CAD build for the part. Positions are in the model's coordinates, mm. A direction names the side the tool comes from. Coordinates: 2 decimals unless noted, no trailing zeros. Loops run counter-clockwise (first coordinate to the right, second up) from the corner with the lowest first, then second, coordinate; pieces in that order, holes last. Notation, with made-up numbers: (-13, 41) -> (6, 41) arc R13 cw to (6, 56) -> close; hole circle Ø8 at (9.5, 40.25). An arc over 180 degrees is marked (long way). Answer as CSV lines item,"result". Start each with the question number.
from build123d import *

# Parameters (mm, degrees)
SKETCH1_R             = 1
BOSS_EXTRUDE1_DEPTH   = 8
BOSS_EXTRUDE1_2_DEPTH = 8
BOSS_EXTRUDE1_3_DEPTH = 8
BOSS_EXTRUDE1_4_DEPTH = 8
SKETCH2_R             = 1.75
BOSS_EXTRUDE2_DEPTH   = 6
SKETCH3_W             = 99
SKETCH3_H             = 63
BOSS_EXTRUDE3_DEPTH   = 2
FILLET1_R             = 2
BOSS_EXTRUDE4_START   = 8
BOSS_EXTRUDE4_DEPTH   = 8
CUT_EXTRUDE1_REACH    = 106.833
SKETCH6_W             = 18
SKETCH6_H             = 7
CUT_EXTRUDE2_REACH    = 83.514
SKETCH8_W             = 18
SKETCH8_H             = 7


with BuildPart() as part:
    # Sketch1 → Boss-Extrude1 (new body)
    with BuildSketch(Plane(origin=(0, 0, 0), x_dir=(1, 0, 0), z_dir=(0, 1, 0))):
        with Locations(Location((-33.5, 25, 0), (0, 0, 270))):
            Circle(SKETCH1_R)
    extrude(amount=BOSS_EXTRUDE1_DEPTH)



with BuildPart() as body_2:
    # Sketch1 → Boss-Extrude1 2 (new body)
    with BuildSketch(Plane(origin=(0, 0, 0), x_dir=(1, 0, 0), z_dir=(0, 1, 0))):
        with Locations(Location((33.5, 25, 0), (0, 0, 270))):
            Circle(SKETCH1_R)
    extrude(amount=BOSS_EXTRUDE1_2_DEPTH)


with BuildPart() as body_3:
    # Sketch1 → Boss-Extrude1 3 (new body)
    with BuildSketch(Plane(origin=(0, 0, 0), x_dir=(1, 0, 0), z_dir=(0, 1, 0))):
        with Locations(Location((-45.75, -25, 0), (0, 0, 270))):
            Circle(SKETCH1_R)
    extrude(amount=BOSS_EXTRUDE1_3_DEPTH)


with BuildPart() as body_4:
    # Sketch1 → Boss-Extrude1 4 (new body)
    with BuildSketch(Plane(origin=(0, 0, 0), x_dir=(1, 0, 0), z_dir=(0, 1, 0))):
        with Locations(Location((43.25, -25, 0), (0, 0, 270))):
            Circle(SKETCH1_R)
    extrude(amount=BOSS_EXTRUDE1_4_DEPTH)


with BuildPart() as part_1:
    add(part.part)

    add(body_2.part)  # Boss-Extrude2 merges body 2

    add(body_3.part)  # Boss-Extrude2 merges body 3

    add(body_4.part)  # Boss-Extrude2 merges body 4
    # Sketch2 → Boss-Extrude2 (add)
    with BuildSketch(Plane(origin=(0, 0, 0), x_dir=(1, 0, 0), z_dir=(0, 1, 0))):
        with Locations(Location((-33.5, 25, 0), (0, 0, 270))):
            Circle(SKETCH2_R)
        with Locations(Location((33.5, 25, 0), (0, 0, 270))):
            Circle(SKETCH2_R)
        with Locations(Location((43.25, -25, 0), (0, 0, 270))):
            Circle(SKETCH2_R)
        with Locations(Location((-45.75, -25, 0), (0, 0, 270))):
            Circle(SKETCH2_R)
    extrude(amount=BOSS_EXTRUDE2_DEPTH)

    # Sketch3 → Boss-Extrude3 (add)
    with BuildSketch(Plane(origin=(0, 0, 0), x_dir=(1, 0, 0), z_dir=(0, 1, 0))):
        with Locations((-1.25, 1.5)):
            Rectangle(SKETCH3_W, SKETCH3_H)
    extrude(amount=BOSS_EXTRUDE3_DEPTH)

    # Fillet1
    fillet1_edges = [part_1.edges().sort_by_distance(p)[0] for p in [
        (-50.75, 1, -33),
        (-50.75, 1, 30),
        (48.25, 1, 30),
        (48.25, 1, -33),
    ]]
    fillet(fillet1_edges, radius=FILLET1_R)

    # Sketch4 → Boss-Extrude4 (add)
    with BuildSketch(Plane(origin=(0, 2, 0), x_dir=(1, 0, 0), z_dir=(0, 1, 0)).offset(BOSS_EXTRUDE4_START)):
        with BuildLine():
            Line((-47.25, -28.5), (44.75, -28.5))
            ThreePointArc((44.75, -28.5), (46.164213562, -27.914213562), (46.75, -26.5))
            Line((46.75, -26.5), (46.75, 32.936491673))
            ThreePointArc((46.75, 32.936491673), (47.83113883, 32.224744871), (48.25, 31))
            Line((48.25, 31), (48.25, -28))
            ThreePointArc((48.25, -28), (47.664213562, -29.414213562), (46.25, -30))
            Line((46.25, -30), (-48.75, -30))
            ThreePointArc((-48.75, -30), (-50.164213562, -29.414213562), (-50.75, -28))
            Line((-50.75, -28), (-50.75, 31))
            ThreePointArc((-50.75, 31), (-50.33113883, 32.224744871), (-49.25, 32.936491673))
            Line((-49.25, 32.936491673), (-49.25, -26.5))
            ThreePointArc((-49.25, -26.5), (-48.664213562, -27.914213562), (-47.25, -28.5))
        make_face()
    extrude(amount=-BOSS_EXTRUDE4_DEPTH)

    # Sketch6 → Cut-Extrude1 (cut, up to next)
    with BuildSketch(Plane.ZY.offset(50.75), mode=Mode.PRIVATE) as cut_extrude1_sk1:
        with Locations((-4.936491673, 6.5)):
            Rectangle(SKETCH6_W, SKETCH6_H)
    cut_extrude1_tool1 = extrude(cut_extrude1_sk1.sketch, amount=-CUT_EXTRUDE1_REACH, mode=Mode.PRIVATE) & part_1.part
    add(cut_extrude1_tool1.solids().sort_by_distance((-50.75, 6.5, -4.936492))[0], mode=Mode.SUBTRACT)

    # Sketch8 → Cut-Extrude2 (cut, up to next)
    with BuildSketch(Plane.XY.offset(30), mode=Mode.PRIVATE) as cut_extrude2_sk1:
        with Locations((-27.25, 6.5)):
            Rectangle(SKETCH8_W, SKETCH8_H)
    cut_extrude2_tool1 = extrude(cut_extrude2_sk1.sketch, amount=-CUT_EXTRUDE2_REACH, mode=Mode.PRIVATE) & part_1.part
    add(cut_extrude2_tool1.solids().sort_by_distance((-27.25, 6.5, 30))[0], mode=Mode.SUBTRACT)


solid = part_1.part
Item 1: Saw through at B-B (z = -2). Write the cut outline in (x, y).
Item 2: Flat gauge pins, fed straight in: pin 1 Ø1 at (x, z) = (43.5, 24.5) entering from +Y; pin 2 Ø1 at (x, y) = (-38, 3) entering from -Z; pin 3 Ø0.8 at (x, y) = (-50, 8) entering from +Z. Where does each tip first touch, or does it go through?
Item 3: Wall check: probe 1 along X at (y, z) = (5, 26); probe 2 along X at (y, z) = (4, 25.5); probe 3 along X at (y, z) = (8, 6.5). Give the ranges that are in metal, low to high.
Item 4: Saw through at A-A (y = 4). Write the cut outline in (x, z), plus the area to 3 significant figures.
Item 5: Two-plate mould, pull along Z, no slides. Class faces 1 (the face through (-2, 0, -2)), 2 (the face through (32, 6, -25)), 3 (the face through (47.68, 5.07, 29.4)): pulls with the +Z half, pulls with the -Z half, needs draft (parallel to the pull), parting line crosses it, or undercut.
Item 6: Which spindle directions (+Z, -Z, +X, -X, +Y, -Y) get a long thin tool onto all of the face, cutting with end or side? Do faces 4 (the face through (-50.75, 2.8, -1.1)), 5 (the face through (43, 8, 25)), 6 (the face through (-33, 8, -25)), 7 (the face through (48.25, 5, -2)), 8 (the face through (-35, 6, -25)). Say none if no direction does.
Item 7: Saw through at D-D (z = 14.5). Write the cut outline in (x, y), plus the area to 3 significant figures.
Item 8: Saw through at C-C (x = 33.5). Write the cut outline in (y, z).
Geometry check:
1,outline,"(-50.75, 0) -> (48.25, 0) -> (48.25, 10) -> (46.75, 10) -> (46.75, 2) -> (-49.25, 2) -> (-49.25, 3) -> (-50.75, 3) -> close"
2,pin 1,"y = 8"
2,pin 2,"z = 28.5"
2,pin 3,"z = 29.81"
3,probe 1,"-50.75 to -49.25, -47.19 to -44.31, 41.81 to 44.69, 46.75 to 48.25"
3,probe 2,"-50.75 to -49.25, -47.43 to -44.07, 41.57 to 44.93, 46.75 to 48.25"
3,probe 3,"-50.75 to -49.25, 46.75 to 48.25"
4,outline,"(-50.75, -31) arc R2 ccw to (-49.25, -32.94) -> (-49.25, -13.94) -> (-50.75, -13.94) -> close; (-50.75, 4.06) -> (-49.25, 4.06) -> (-49.25, 26.5) arc R2 cw to (-47.25, 28.5) -> (-36.25, 28.5) -> (-36.25, 30) -> (-48.75, 30) arc R2 ccw to (-50.75, 28) -> close; circle Ø3.5 at (-45.75, 25); circle Ø3.5 at (-33.5, -25); (-18.25, 28.5) -> (44.75, 28.5) arc R2 cw to (46.75, 26.5) -> (46.75, -32.94) arc R2 ccw to (48.25, -31) -> (48.25, 28) arc R2 ccw to (46.25, 30) -> (-18.25, 30) -> close; circle Ø3.5 at (33.5, -25); circle Ø3.5 at (43.25, 25)"
4,area,"316 mm2"
5,face 1,"needs draft"
5,face 2,"undercut"
5,face 3,"pulls with the +Z half"
6,face 4,"+Z, -Z, -X, +Y, -Y"
6,face 5,"-Z, +Y"
6,face 6,"+Z, -Z, +Y"
6,face 7,"+Z, -Z, +X, +Y, -Y"
6,face 8,"+Y"
7,outline,"(-50.75, 0) -> (48.25, 0) -> (48.25, 10) -> (46.75, 10) -> (46.75, 2) -> (-49.25, 2) -> (-49.25, 10) -> (-50.75, 10) -> close"
7,area,"222 mm2"
8,outline,"(0, -33) -> (2, -33) -> (2, -26.75) -> (6, -26.75) -> (6, -26) -> (8, -26) -> (8, -24) -> (6, -24) -> (6, -23.25) -> (2, -23.25) -> (2, 28.5) -> (10, 28.5) -> (10, 30) -> (0, 30) -> close"
